Autodesk Inventor part; units mm, degrees
ref_plane "YZ Plane" through (0, 0, 0) normal (1, 0, 0) x (0, 1, 0)
ref_plane "XZ Plane" through (0, 0, 0) normal (0, 1, 0) x (-1, 0, 0)
ref_plane "XY Plane" through (0, 0, 0) normal (0, 0, 1) x (1, 0, 0)
sketch "Sketch1" plane through (0, 0, 0) normal (1, 0, 0) x (0, 1, 0)
  line L0 (6.35, 0) -> (6.35, 3.175)
  line L1 (6.35, 3.175) -> (4.7137, 1.7526)
  line L2 (4.7137, 1.7526) -> (0, 1.7526)
  line L3 (0, 1.7526) -> (0, 0)
  line L4 (0, 0) -> (6.35, 0)
  line L5 (6.35, 0) -> (6.35, -3.175) construction
  line L6 (6.35, -3.175) -> (4.7137, -1.7526) construction
  line L7 (4.7137, -1.7526) -> (0, -1.7526) construction
  line L8 (0, -1.7526) -> (0, 0) construction
  dimension "d0" = 6.35
  dimension "d1" = 3.5052
  dimension "d2" = 82
  dimension "d3" = 6.35
revolve "Revolution1" add sketch "Sketch1" angle 360 about axis through (0, 0, 0) along (0, 1, 0)
sketch "Sketch2" plane through (0, 0, 0) normal (1, 0, 0) x (0, 1, 0)
  line L0 (4.7137, -1.7526) -> (4.7137, 1.7526) construction
  line L1 (6.35, -3.175) -> (6.35, 3.175) construction
  line L2 (6.35, -3.175) -> (6.35, 3.175)
  line L3 (6.35, 0.635) -> (5.461, 0.635)
  line L4 (5.461, 0.635) -> (5.461, -0.635)
  line L5 (5.461, -0.635) -> (6.35, -0.635)
  line L6 (6.35, -0.635) -> (6.35, 0.635)
  line L7 (6.35, 0) -> (4.7137, 0) construction
  point P0 (0, 0)
  dimension "d5" = 1.27
  dimension "d6" = 0.889
extrude "Extrusion1" cut sketch "Sketch2" along normal through all both and the other way through all
chamfer "Chamfer1" distance 0.381 angle 45 1 edges at (0, 0, -1.7526)
thread "Thread1"
properties part number "6-32x0.25 Slotted Flathead" material "Stainless Steel, 440C"
Part model, mm, in its own coordinate system. A direction names the side the tool comes from. Round coordinates to 2 decimals unless told otherwise and drop trailing zeros. Loops run counter-clockwise (first coordinate to the right, second up) from the corner with the lowest first, then second, coordinate; pieces in that order, holes last. Notation, with made-up numbers: (-15.75, 28.5) - (33.25, 28.5) arc R18 cw to (33.25, 60.5) - close; hole circle Ø4 at (84, 5.5). An arc over 180 degrees is marked (long way). Answer as a JSON object with one key per item and string values.
Item 1: Pin check, flat tips, straight feed: pin 1 (1.5 mm diameter, centred on y = 3, z = 1.5, fed in from -X); pin 2 (1 mm diameter, centred on y = 2.5, z = 1.5, fed in from -X); pin 3 (1 mm diameter, centred on x = -1, y = 6, fed in from +Z). Stop position of each tip, or through.
Output:
{"pin 1": "x = -1.58", "pin 2": "x = -1.44", "pin 3": "z = 3.11"}
Item 2: Tool access for faces 4 (the face through (0, 6, -0.635)), 5 (the face through (-2, 5, 0)): list every direction of +Z, -Z, +X, -X, +Y, -Y with a clear straight run to the whole face (end or side of a thin tool).
Output:
{"face 4": "+X, -X, +Y", "face 5": "-Y"}
Item 3: Band-saw the part on C-C on y = 4. List the corners of the cut face in (x, z), plus the area to 3 significant figures.
Output:
{"outline": "circle Ø3.51 at (0, 0)", "area": "9.65 mm2"}
Item 4: Band-saw the part on B-B on x = 0. List the corners of the cut face in (y, z) (3 decimals).
Output:
{"outline": "(0, -1.372) - (0.381, -1.753) - (4.714, -1.753) - (6.35, -3.175) - (6.35, -0.635) - (5.461, -0.635) - (5.461, 0.635) - (6.35, 0.635) - (6.35, 3.175) - (4.714, 1.753) - (0.381, 1.753) - (0, 1.372) - close"}
Item 5: Pull direction Z, two halves, no side cores. Call faces 1 (the face through (-0.53, 2.52, 1.67)), 2 (the face through (0, 0, 0)), 3 (the face through (0, 5.461, 0)): pulls with the +Z half, pulls with the -Z half, needs draft (parallel to the pull), parting line crosses it, or undercut.
Output:
{"face 1": "parting line crosses it", "face 2": "needs draft", "face 3": "undercut"}
Item 6: Band-saw the part on A-A on z = 0. List the corners of the cut face in (x, y).
Output:
{"outline": "(-2.4, 5.46) - (-1.75, 4.71) - (-1.75, 0.38) - (-1.37, 0) - (1.37, 0) - (1.75, 0.38) - (1.75, 4.71) - (2.4, 5.46) - close"}
Item 7: Wall check: L1, parallel to X at y = 4, z = 0; L2, parallel to Z at x = 0.75, y = 6.25 (3 decimals); L3, parallel to Z at x = 0.5, y = 5.5 (3 decimals). Give the ranges that are in metal, low to high.
Output:
{"L1": "-1.75 to 1.75", "L2": "-2.996 to -0.635, 0.635 to 2.996", "L3": "-2.384 to -0.635, 0.635 to 2.384"}
